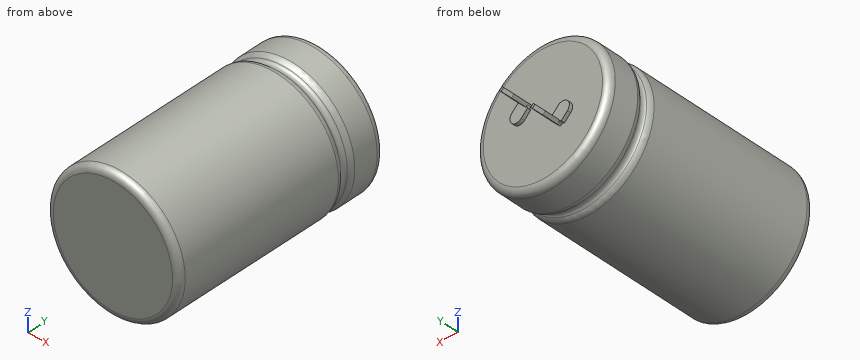
```python
from build123d import *
from OCP.BRepFilletAPI import BRepFilletAPI_MakeChamfer

# Parameters (mm, degrees)
FILLET_1_R      = 1.5
EXTRUDE_4_DEPTH = 6.3
EXTRUDE_5_DEPTH = 0.8
CHAMFER_2_SIZE  = 2
CHAMFER_2_SIZE2 = 0.727940469
FILLET_4_R      = 0.5


with BuildPart() as part:
    # Эскиз2 → Повернуть1 (revolve)
    with BuildSketch(Plane.XY, mode=Mode.PRIVATE) as revolve_1_sk:
        with BuildLine():
            Line((0, 0), (-15, 0))
            Line((-15, 0), (-15, 40))
            ThreePointArc((-15, 40), (-14, 41), (-15, 42))
            Line((-15, 42), (-15, 50))
            Line((-15, 50), (0, 50))
            Line((0, 50), (0, 0))
        make_face()
    revolve(revolve_1_sk.sketch.rotate(Axis((0, 0, 0), (0, 1, 0)), 270), axis=Axis((0, 0, 0), (0, 1, 0)))

    # Скругление1
    fillet_1_edges = [part.edges().sort_by_distance(p)[0] for p in [
        (0, 0, 15),
        (0, 40, 15),
        (0, 42, 15),
        (0, 50, 15),
    ]]
    fillet(fillet_1_edges, radius=FILLET_1_R)

    # Эскиз3 → Бобышка-Вытянуть4 (add)
    with BuildSketch(Plane(origin=(0, 50, 0), x_dir=(1, 0, 0), z_dir=(0, 1, 0))):
        Polygon((-4.5254834, 3.959797975), (-3.111269837, 2.545584412), (-2.545584412, 3.111269837), (-3.959797975, 4.5254834), align=None)
        Polygon((3.959797975, -4.5254834), (2.545584412, -3.111269837), (3.111269837, -2.545584412), (4.5254834, -3.959797975), align=None)
    extrude(amount=EXTRUDE_4_DEPTH)

    # Эскиз5 → Бобышка-Вытянуть5 (add)
    with BuildSketch(Plane(origin=(0, 50, 0), x_dir=(1, 0, 0), z_dir=(0, 1, 0))):
        with BuildLine():
            Line((-2.757716447, 2.192031022), (-4.87903679, 4.313351365))
            Line((-4.87903679, 4.313351365), (-6.293250353, 2.899137803))
            ThreePointArc((-6.293250353, 2.899137803), (-6.293250353, 0.777817459), (-4.171930009, 0.777817459))
            Line((-4.171930009, 0.777817459), (-2.757716447, 2.192031022))
        make_face()
        with BuildLine():
            Line((4.87903679, -4.313351365), (2.757716447, -2.192031022))
            Line((2.757716447, -2.192031022), (4.171930009, -0.777817459))
            ThreePointArc((4.171930009, -0.777817459), (6.293250353, -0.777817459), (6.293250353, -2.899137803))
            Line((6.293250353, -2.899137803), (4.87903679, -4.313351365))
        make_face()
    extrude(amount=EXTRUDE_5_DEPTH)

    # Фаска2: one chamfer whose edges measure the first distance from different faces: ONE call of the kernel's chamfer builder (chamfer() names one face for all edges)
    chamfer_2_edges_1 = [part.edges().sort_by_distance(p)[0] for p in [
        (-4.242640687, 56.3, -4.242640687),
    ]]
    chamfer_2_side_1 = [part.faces().sort_by_distance(p)[0] for p in [
        (-4.242640687, 53.15, -4.242640687),
    ]]
    chamfer_2_edges_2 = [part.edges().sort_by_distance(p)[0] for p in [
        (-2.828427125, 56.3, -2.828427125),
    ]]
    chamfer_2_side_2 = [part.faces().sort_by_distance(p)[0] for p in [
        (-2.828427125, 53.15, -2.828427125),
    ]]
    chamfer_2_edges_3 = [part.edges().sort_by_distance(p)[0] for p in [
        (4.242640687, 56.3, 4.242640687),
    ]]
    chamfer_2_side_3 = [part.faces().sort_by_distance(p)[0] for p in [
        (4.242640687, 53.15, 4.242640687),
    ]]
    chamfer_2_edges_4 = [part.edges().sort_by_distance(p)[0] for p in [
        (2.828427125, 56.3, 2.828427125),
    ]]
    chamfer_2_side_4 = [part.faces().sort_by_distance(p)[0] for p in [
        (2.828427125, 53.15, 2.828427125),
    ]]
    chamfer_2 = BRepFilletAPI_MakeChamfer(part.part.solid().wrapped)
    for e in chamfer_2_edges_1:
        chamfer_2.Add(CHAMFER_2_SIZE, CHAMFER_2_SIZE2, e.wrapped, chamfer_2_side_1[0].wrapped)  # the first distance lies on this face
    for e in chamfer_2_edges_2:
        chamfer_2.Add(CHAMFER_2_SIZE, CHAMFER_2_SIZE2, e.wrapped, chamfer_2_side_2[0].wrapped)  # the first distance lies on this face
    for e in chamfer_2_edges_3:
        chamfer_2.Add(CHAMFER_2_SIZE, CHAMFER_2_SIZE2, e.wrapped, chamfer_2_side_3[0].wrapped)  # the first distance lies on this face
    for e in chamfer_2_edges_4:
        chamfer_2.Add(CHAMFER_2_SIZE, CHAMFER_2_SIZE2, e.wrapped, chamfer_2_side_4[0].wrapped)  # the first distance lies on this face
    add(Compound.cast(chamfer_2.Shape()), mode=Mode.REPLACE)

    # Скругление4
    fillet_4_edges = [part.edges().sort_by_distance(p)[0] for p in [
        (3.111269837, 50.4, 2.545584412),
        (4.5254834, 50.4, 3.959797975),
        (-4.5254834, 50.4, -3.959797975),
        (-3.111269837, 50.4, -2.545584412),
    ]]
    fillet(fillet_4_edges, radius=FILLET_4_R - 0.0001)  # a hair under: the kernel refuses the full size


solid = part.part
```
Input: part model. Units: mm. Frame: model coordinates. Round coordinates to 2 decimals unless told otherwise and drop trailing zeros. Loops run counter-clockwise (first coordinate to the right, second up) from the corner with the lowest first, then second, coordinate; pieces in that order, holes last. Notation, with made-up numbers: M 59.25,42 L 76.25,42 A26 cw 76.25,70 Z; hole C -38,-32 d4. An arc over 180 degrees is marked long. Answer in a Markdown table with one row per item. Add a question column.
1. Ray query, probe 1 along Z at (x, y) = (-0.5, 9); probe 2 along Y at (x, z) = (-4, 3.5); probe 3 along Y at (x, z) = (10, 10). Return the intervals inside material, ascending.
2. Contact query for flat-ended pins moving along their axis: pin 1 (10 mm diameter, centred on x = -7.5, y = 24.5, fed in from +Z); pin 2 (2 mm diameter, centred on x = -5, z = -2, fed in from +Y); pin 3 (10 mm diameter, centred on x = 1, z = -0.5, fed in from -Y); pin 4 (4 mm diameter, centred on x = -8, y = 15, fed in from -Z). Output: stop coordinate, or through.
3. Section A-A (y = 33.5). Output: boundary loops of the cut face in (x, z).
Values follow:
| question | item | result |
|---|---|---|
| 1 | probe 1 | -14.99 to 14.99 |
| 1 | probe 2 | 0 to 50 |
| 1 | probe 3 | 0.14 to 40.49, 41.51 to 49.86 |
| 2 | pin 1 | z = 14.79 |
| 2 | pin 2 | y = 50.8 |
| 2 | pin 3 | y = 0 |
| 2 | pin 4 | z = -13.75 |
| 3 | outline | C 0,0 d30 |
